from build123d import *

# Parameters (mm, degrees)
SKETCH015_W     = 38.1
SKETCH015_H     = 5
PAD002_DEPTH    = 150
SKETCH016_R     = 4.25
POCKET004_DEPTH = 5.001
SKETCH017_R     = 8.25
POCKET005_DEPTH = 3
SKETCH018_R     = 1.7
POCKET006_DEPTH = 5.001
SKETCH019_R     = 2.925
POCKET007_DEPTH = 3.5


with BuildPart() as part:
    # Sketch015 → Pad002 (new body)
    with BuildSketch(Plane.XZ.offset(75)):
        with Locations((19.05, 2.5)):
            Rectangle(SKETCH015_W, SKETCH015_H)
    extrude(amount=-PAD002_DEPTH)

    # Sketch016 → Pocket004 (cut, through all)
    with BuildSketch(Plane.XY):
        with Locations((19.05, 61.875)):
            Circle(SKETCH016_R)
        with Locations((19.05, -61.875)):
            Circle(SKETCH016_R)
    extrude(amount=POCKET004_DEPTH, mode=Mode.SUBTRACT)

    # Sketch017 → Pocket005 (cut)
    with BuildSketch(Plane.XY.offset(5)):
        with Locations((19.05, 61.875)):
            Circle(SKETCH017_R)
        with Locations((19.05, -61.875)):
            Circle(SKETCH017_R)
    extrude(amount=-POCKET005_DEPTH, mode=Mode.SUBTRACT)

    # Sketch018 → Pocket006 (cut, through all)
    with BuildSketch(Plane.XY):
        with Locations((9.525, 25.4)):
            Circle(SKETCH018_R)
        with Locations((28.575, 25.4)):
            Circle(SKETCH018_R)
        with Locations((9.525, -25.4)):
            Circle(SKETCH018_R)
        with Locations((28.575, -25.4)):
            Circle(SKETCH018_R)
    extrude(amount=POCKET006_DEPTH, mode=Mode.SUBTRACT)

    # Sketch019 → Pocket007 (cut)
    with BuildSketch(Plane.XY):
        with Locations((9.525, 25.4)):
            Circle(SKETCH019_R)
        with Locations((28.575, 25.4)):
            Circle(SKETCH019_R)
        with Locations((9.525, -25.4)):
            Circle(SKETCH019_R)
        with Locations((28.575, -25.4)):
            Circle(SKETCH019_R)
    extrude(amount=POCKET007_DEPTH, mode=Mode.SUBTRACT)


with BuildPart() as part_1:
    # Body001 placement: moved
    add(part.part.moved(Location((0, 0, -27))))


solid = part_1.part
Input: part model. Units: mm. Frame: model coordinates. A direction names the side the tool comes from. Coordinates: 2 decimals unless noted, no trailing zeros. Order: outer loops, then holes, each group sorted by start corner. A loop starts at its lowest first (then second) coordinate and runs counter-clockwise, first axis right, second up.
1. Access query for faces 1 (the cylindrical face through (23.49, 68.83, -23.48)), 2 (the flat face through (11, -27, -23.5)), 3 (the cylindrical face through (9.16, 23.74, -22.76)). Directions: +Z, -Z, +X, -X, +Y, -Y. A direction counts if a zero-diameter tool reaches every point of the face in a straight line with its end or side. Return the directions, or none.
Checked values:
face 1: +Z
face 2: -Z
face 3: +Z, -Z
2. Draft query along X for faces 4 (the flat face through (11, 24, -23.5)), 5 (the flat face through (19, -1, -22)). Return one class per face: +X half, -X half, draft (parallel to the pull), parting line (faces both ways), or undercut.
Checked values:
face 4: undercut
face 5: draft
3. Cut plane A-A, the plane x = 19.05. Return loops of the section in (y, z) (3 decimals), plus the area to 3 significant figures.
Checked values:
outline: (-75, -27) - (-66.125, -27) - (-66.125, -25) - (-70.125, -25) - (-70.125, -22) - (-75, -22) - close; (-57.625, -27) - (57.625, -27) - (57.625, -25) - (53.625, -25) - (53.625, -22) - (-53.625, -22) - (-53.625, -25) - (-57.625, -25) - close; (66.125, -27) - (75, -27) - (75, -22) - (70.125, -22) - (70.125, -25) - (66.125, -25) - close
area: 617 mm2
4. Cut plane C-C, the plane z = -22.75. Return loops of the section in (x, y) (3 decimals).
Checked values:
outline: (0, -75) - (38.1, -75) - (38.1, 75) - (0, 75) - close; hole circle Ø3.4 at (9.525, -25.4); hole circle Ø3.4 at (9.525, 25.4); hole circle Ø16.5 at (19.05, -61.875); hole circle Ø16.5 at (19.05, 61.875); hole circle Ø3.4 at (28.575, -25.4); hole circle Ø3.4 at (28.575, 25.4)
5. Ray query, line 1 along Y through (x, z) = (29, -24); line 2 along Y through (x, z) = (19.05, -26.2) (3 decimals); line 3 along X through (y, z) = (25.4, -23.05) (3 decimals). Return the intervals inside material, ascending.
Checked values:
line 1: y = -75 to -28.29, -22.51 to 22.51, 28.29 to 75
line 2: y = -75 to -66.125, -57.625 to 57.625, 66.125 to 75
line 3: x = 0 to 7.825, 11.225 to 26.875, 30.275 to 38.1
6. Contact query for flat-ended pins moving along their axis: P1, Ø6.5, axis at x = 8, y = -26, coming from the -Z side; P2, Ø5, axis at x = 19.5, y = 66, coming from the +Z side; P3, Ø4, axis at x = 28.575, y = 25.4, coming from the -Z side. Output: stop coordinate, or through.
Checked values:
P1: stops at z = -27
P2: stops at z = -25
P3: stops at z = -23.5
7. Cut plane B-B, the plane y = -25.4. Return loops of the section in (x, z) (3 decimals).
Checked values:
outline: (0, -27) - (6.6, -27) - (6.6, -23.5) - (7.825, -23.5) - (7.825, -22) - (0, -22) - close; (11.225, -23.5) - (12.45, -23.5) - (12.45, -27) - (25.65, -27) - (25.65, -23.5) - (26.875, -23.5) - (26.875, -22) - (11.225, -22) - close; (30.275, -23.5) - (31.5, -23.5) - (31.5, -27) - (38.1, -27) - (38.1, -22) - (30.275, -22) - close
